Design review of the part built by this model. Coordinates are the model's own, in mm. Face numbers are marked on the shaded views. A direction names the side the tool comes from. Round coordinates to 2 decimals unless told otherwise and drop trailing zeros. Loops run counter-clockwise (first coordinate to the right, second up) from the corner with the lowest first, then second, coordinate; pieces in that order, holes last. Notation, with made-up numbers: (33, -24.75) - (71, -24.75) arc R7 cw to (71, -17.75) - close; hole circle Ø9 at (67.25, 63.25). An arc over 180 degrees is marked (long way). Return JSON: item names as keys, results as strings. Group by question number.
(1) Clearance check with a flat-ended pin moving along its axis: pin 1 (5 mm diameter, centred on y = -10, z = 1.5, fed in from +X). State where the tip first meets the part, or that it passes through.
(2) We need section B-B, the plane z = 1.75. Give the number of separate pieces and of enclosed holes in the cut face, and give its area (3 significant figures).
(3) For the marked faces 1 and 2, list the 3-axis set-ups (+Z, -Z, +X, -X, +Y, -Y) from which the entire face can be reached by the end or side of a thin tool; tool diameter is ignored.
(4) Wall thickness on L1, parallel to Y at x = 0, z = -1.75; L2, parallel to X at y = -3, z = -2.5; L3, parallel to X at y = 19, z = -1: over which ranges is each line inside the solid? List them lowest first. Write a range as [from, to].
(5) We need section A-A, the plane y = -2. Write out the cut boundary in (x, z) (3 decimals), and give its area (3 significant figures).
(6) We need section C-C, the plane x = -77.5. Write out the cut boundary in (y, z) (3 decimals), and give its area (3 significant figures).
(7) We need section D-D, the plane x = -53.76. Write out the cut boundary in (y, z) (3 decimals).
(8) The part is to be moulded in two halves that separate along Y. For the marked faces 3, 4, 5 and 6, say which applies: pulls with the +Y half, pulls with the -Y half, needs draft (parallel to the pull), parting line crosses it, or undercut.
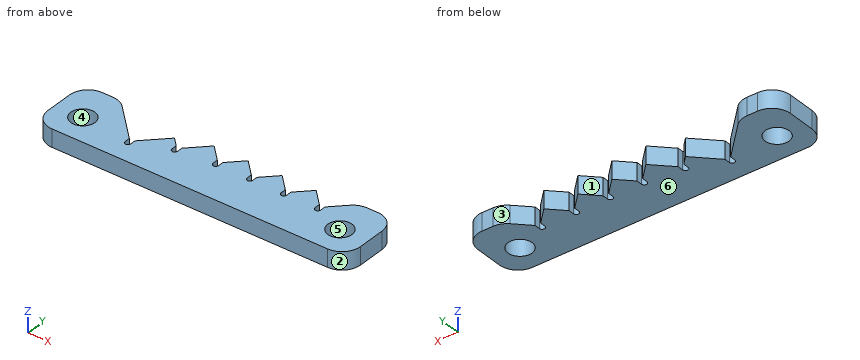
from build123d import *

# Parameters (mm, degrees)
CROQUIS9_R              = 6.5
SALIENTE_EXTRUIR1_DEPTH = 4.765
REDONDEO1_R             = 10


with BuildPart() as part:
    # Croquis9 → Saliente-Extruir1 (new, symmetric)
    with BuildSketch(Plane.XY):
        with BuildLine():
            Line((-5, 20), (-15.5, 9.5))
            Line((-15.5, 9.5), (-15.5, 6.5))
            ThreePointArc((-15.5, 6.5), (-17, 5), (-18.5, 6.5))
            Line((-18.5, 6.5), (-18.5, 9.5))
            Line((-18.5, 9.5), (-26.19, 17.19))
            Line((-26.19, 17.19), (-33.88, 9.5))
            Line((-33.88, 9.5), (-33.88, 6.5))
            ThreePointArc((-33.88, 6.5), (-35.38, 5), (-36.88, 6.5))
            Line((-36.88, 6.5), (-36.88, 9.5))
            Line((-36.88, 9.5), (-44.57, 17.19))
            Line((-44.57, 17.19), (-52.26, 9.5))
            Line((-52.26, 9.5), (-52.26, 6.5))
            ThreePointArc((-52.26, 6.5), (-53.76, 5), (-55.26, 6.5))
            Line((-55.26, 6.5), (-55.26, 9.5))
            Line((-55.26, 9.5), (-62.95, 17.19))
            Line((-62.95, 17.19), (-70.64, 9.5))
            Line((-70.64, 9.5), (-70.64, 6.5))
            ThreePointArc((-70.64, 6.5), (-72.14, 5), (-73.64, 6.5))
            Line((-73.64, 6.5), (-73.64, 9.5))
            Line((-73.64, 9.5), (-81.33, 17.19))
            Line((-81.33, 17.19), (-91.169058454, 7.350941546))
            Line((-91.169058454, 7.350941546), (-91.169058454, 4.350941546))
            ThreePointArc((-91.169058454, 4.350941546), (-92.669058454, 2.850941546), (-94.169058454, 4.350941546))
            Line((-94.169058454, 4.350941546), (-94.169058454, 7.350941546))
            Line((-94.169058454, 7.350941546), (-98.364058454, 11.545941546))
            Line((-98.364058454, 11.545941546), (-110.41, -0.5))
            Line((-110.41, -0.5), (-110.41, -3.5))
            ThreePointArc((-110.41, -3.5), (-111.91, -5), (-113.41, -3.5))
            Line((-113.41, -3.5), (-113.41, -0.5))
            Line((-113.41, -0.5), (-133.91, 20))
            Line((-133.91, 20), (-153.91, 20))
            Line((-153.91, 20), (-153.91, -15))
            Line((-153.91, -15), (15, -15))
            Line((15, -15), (15, 20))
            Line((15, 20), (-5, 20))
        make_face()
        with Locations((-138.91, 0)):
            Circle(CROQUIS9_R, mode=Mode.SUBTRACT)
        Circle(CROQUIS9_R, mode=Mode.SUBTRACT)
    extrude(amount=SALIENTE_EXTRUIR1_DEPTH, both=True)

    # Redondeo1
    redondeo1_edges = [part.edges().sort_by_distance(p)[0] for p in [
        (15, 20, 0),
        (15, -15, 0),
        (-153.91, -15, 0),
        (-153.91, 20, 0),
        (-133.91, 20, 0),
        (-5, 20, 0),
    ]]
    fillet(redondeo1_edges, radius=REDONDEO1_R)


solid = part.part
Solutions:
{
 "1": {"pin 1": "x = 14.68"},
 "2": {"separate pieces": "1", "enclosed holes": "2", "area": "4,340 mm^2"},
 "3": {"face 1": "+Z, -Z, +Y", "face 2": "+Z, -Z, +X, -Y"},
 "4": {"L1": "[-15, -6.5], [6.5, 20]", "L2": "[-153.91, -144.68], [-133.14, -113.41], [-110.41, -5.77], [5.77, 15]", "L3": "[-148.27, -133.69], [-5.22, 9.36]"},
 "5": {"outline": "(-153.91, -4.765) - (-145.095, -4.765) - (-145.095, 4.765) - (-153.91, 4.765) - close; (-132.725, -4.765) - (-113.41, -4.765) - (-113.41, 4.765) - (-132.725, 4.765) - close; (-110.41, -4.765) - (-6.185, -4.765) - (-6.185, 4.765) - (-110.41, 4.765) - close; (6.185, -4.765) - (15, -4.765) - (15, 4.765) - (6.185, 4.765) - close", "area": "1,350 mm^2"},
 "6": {"outline": "(-15, -4.765) - (13.36, -4.765) - (13.36, 4.765) - (-15, 4.765) - close", "area": "270 mm^2"},
 "7": {"outline": "(-15, -4.765) - (5, -4.765) - (5, 4.765) - (-15, 4.765) - close"},
 "8": {"face 3": "pulls with the +Y half", "face 4": "undercut", "face 5": "undercut", "face 6": "needs draft"}
}
